Build history of the part. All positions in model axes, mm. Give positions to 0.01 mm unless a question says otherwise; leave off trailing zeros. Order: outer loops, then holes, each group sorted by start corner. A loop starts at its lowest first (then second) coordinate and runs counter-clockwise, first axis right, second up. Notation, with made-up numbers: (4.5, -27.5) - (34.5, -27.5) arc R24 cw to (34.5, 11.5) - close; hole circle Ø10 at (-39, 12.25). An arc over 180 degrees is marked (long way). Use a Markdown table: item, result.
Autodesk Inventor part; units mm, degrees
ref_plane "YZ Plane" through (0, 0, 0) normal (1, 0, 0) x (0, 1, 0)
ref_plane "XZ Plane" through (0, 0, 0) normal (0, 1, 0) x (-1, 0, 0)
ref_plane "XY Plane" through (0, 0, 0) normal (0, 0, 1) x (1, 0, 0)
sketch "Sketch1" plane through (0, 0, 0) normal (0, 1, 0) x (-1, 0, 0)
  line L0 (0, 0) -> (0, 190.5)
  line L1 (0, 190.5) -> (-19.3142, 47.0141)
  line L2 (-19.3142, 47.0141) -> (0, 0)
  line L3 (8.2867, -3.4607) -> (-3.4607, -8.2867)
  line L4 (-3.4607, -8.2867) -> (-25.8344, 46.1749)
  line L5 (-25.8344, 46.1749) -> (-14.0871, 51.0009)
  line L6 (-14.0871, 51.0009) -> (8.2867, -3.4607)
  line L7 (-5.4461, 197.6404) -> (7.1404, 195.9461)
  line L8 (7.1404, 195.9461) -> (-13.2479, 44.4807)
  line L9 (-13.2479, 44.4807) -> (-25.8344, 46.1749)
  line L10 (-25.8344, 46.1749) -> (-5.4461, 197.6404)
  circle A0 centre (0, 0) radius 2.5797
  circle A1 centre (-19.3142, 47.0141) radius 2.5797
  circle A2 centre (0, 190.5) radius 2.5797
  point P0 (0.8471, 196.7932)
  point P1 (2.413, -5.8737)
  point P2 (-12.7939, 47.8532)
  dimension "d0" = 150
  dimension "d1" = 190.5
  dimension "d2" = 144.78
  dimension "d3" = 12.7
  dimension "d4" = 5.1594
  dimension "d5" = 6.35
  dimension "d6" = 6.35
extrude "Extrusion1" add sketch "Sketch1" along normal blind 3.175 contours A0 L2 A1 L9 L8 L6 L0 | L0 L6 L3 L4 L9 A1 L2 A0 | A1 L9 L2 | L2 L9 A1 | L8 L6 L5 A1 L1 A2 L0 | L0 A2 L1 A1 L5 L10 L7 L8 | L8 L9 A1 L5 L6 | L9 A1 L5 L1 L2 | L2 L1 L5 A1 L9 | L9 L5 A1 | A1 L1 L5 | L5 L1 A1
fillet "Fillet1" radius 3.175 6 edges at (-7.1404, 1.5875, 195.9461) (5.4461, 1.5875, 197.6404) (25.8344, 1.5875, 46.1749) (12.7939, 1.5875, 47.8532) (3.4607, 1.5875, -8.2867) (-8.2867, 1.5875, -3.4607)
properties part number "PB IN"
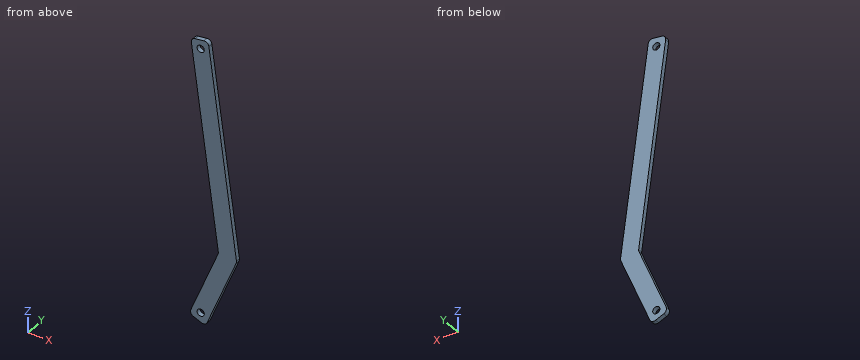
1) Slice it at B-B (z = 190.5). Write the cut outline in (x, y) (3 decimals).
Computed:
| item | result |
|---|---|
| outline | (-6.407, 0) - (-2.58, 0) - (-2.58, 3.175) - (-6.407, 3.175) - close; (2.58, 0) - (6.407, 0) - (6.407, 3.175) - (2.58, 3.175) - close |
2) Slice it at C-C (x = 15). Write the cut outline in (y, z) (3 decimals).
Computed:
| item | result |
|---|---|
| outline | (0, 19.802) - (3.175, 19.802) - (3.175, 126.664) - (0, 126.664) - close |
3) Wall check: line 1 (X direction, y = 1.1, z = 190.5); line 2 (X direction, y = 2.25, z = 0) (3 decimals); line 3 (X direction, y = 2.9, z = 159.5). Give the ranges that are in metal, low to high. Write a range as from..to.
Computed:
| item | result |
|---|---|
| line 1 | x = -6.41..-2.58, 2.58..6.41 |
| line 2 | x = -6.865..-2.58, 2.58..6.865 |
| line 3 | x = -2.23..10.58 |
4) Slice it at D-D (z = 66.5). Write the cut outline in (x, y) (1 decimal).
Computed:
| item | result |
|---|---|
| outline | (10.3, 0) - (23.1, 0) - (23.1, 3.2) - (10.3, 3.2) - close |
5) Slice it at A-A (y = 0.95). State how many separate pieces and enclosed holes the cut face has, and give its area (3 significant figures).
Computed:
| item | result |
|---|---|
| separate pieces | 1 |
| enclosed holes | 2 |
| area | 2,600 mm² |
6) Pin check, flat tips, straight feed: P1, Ø1.5, axis at x = 10.5, y = 1, coming from the -Z side; P2, Ø1, axis at y = 2.5, z = 118, coming from the +X side. Stop position of each tip, or through.
Computed:
| item | result |
|---|---|
| P1 | stops at z = 7.02 |
| P2 | stops at x = 16.23 |
